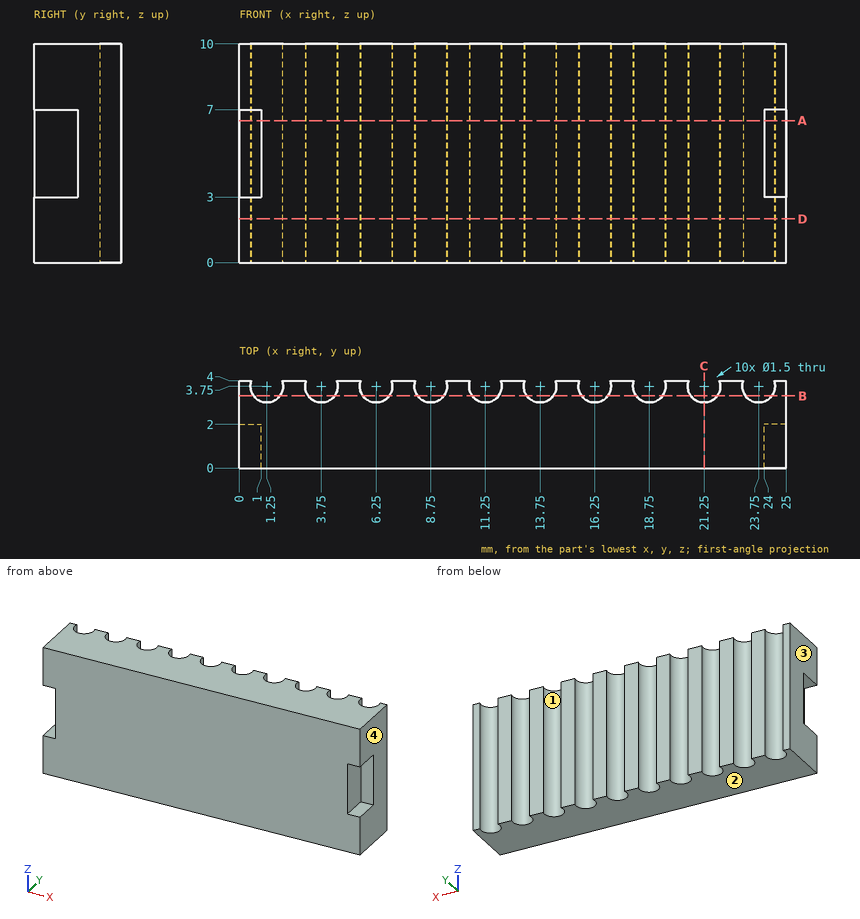
Can you work these out from the drawing? Everything is in mm from the part's minimum corner. Coordinates: 2 decimals unless noted, no trailing zeros. Write each loop counter-clockwise with the first axis right and the second up, starting at its lowest first coordinate (ties: lowest second). Pieces come first, ordered by that corner, then holes. Notation, with made-up numbers: (83.25, -18.5) -> (87.25, -18.5) arc R21 cw to (87.25, -0.5) -> close; hole circle Ø11 at (24.5, 20.25). An arc over 180 degrees is marked (long way). Write each question's results on one line, items separated by ' | '. Start each with the question number.
Q1. Imagine slicing it at A-A (z = 6.5). Write out the boundary of the cut face in (x, y), then the cut area to 3 significant figures.
Q2. Imagine slicing it at D-D (z = 2). Write out the boundary of the cut face in (x, y).
Q3. We'd pull the mould along X, two halves only. Please class the marked faces 1, 2, 3 and 4: +X half, -X half, draft (parallel to the pull), parting line (faces both ways), or undercut.
Q4. Imagine slicing it at B-B (y = 3.3). State how many separate pieces and enclosed holes the cut face has, then the cut area to 3 significant figures.
Q5. Imagine slicing it at C-C (x = 21.25). Write out the boundary of the cut face in (y, z).
Q6. If I drill on probe 1 along Y at (x, z) = (21.5, 1.5); probe 2 along Y at (x, z) = (11.75, 8.5), over which ranges is the centre line in solid material (lowest first)?
Taken from the geometry:
1) outline: (0, 2) -> (1, 2) -> (1, 0) -> (24, 0) -> (24, 2) -> (25, 2) -> (25, 4) -> (24.46, 4) arc R0.75 cw (long way) to (23.04, 4) -> (21.96, 4) arc R0.75 cw (long way) to (20.54, 4) -> (19.46, 4) arc R0.75 cw (long way) to (18.04, 4) -> (16.96, 4) arc R0.75 cw (long way) to (15.54, 4) -> (14.46, 4) arc R0.75 cw (long way) to (13.04, 4) -> (11.96, 4) arc R0.75 cw (long way) to (10.54, 4) -> (9.46, 4) arc R0.75 cw (long way) to (8.04, 4) -> (6.96, 4) arc R0.75 cw (long way) to (5.54, 4) -> (4.46, 4) arc R0.75 cw (long way) to (3.04, 4) -> (1.96, 4) arc R0.75 cw (long way) to (0.54, 4) -> (0, 4) -> close | area: 83.5 mm^2
2) outline: (0, 0) -> (25, 0) -> (25, 4) -> (24.46, 4) arc R0.75 cw (long way) to (23.04, 4) -> (21.96, 4) arc R0.75 cw (long way) to (20.54, 4) -> (19.46, 4) arc R0.75 cw (long way) to (18.04, 4) -> (16.96, 4) arc R0.75 cw (long way) to (15.54, 4) -> (14.46, 4) arc R0.75 cw (long way) to (13.04, 4) -> (11.96, 4) arc R0.75 cw (long way) to (10.54, 4) -> (9.46, 4) arc R0.75 cw (long way) to (8.04, 4) -> (6.96, 4) arc R0.75 cw (long way) to (5.54, 4) -> (4.46, 4) arc R0.75 cw (long way) to (3.04, 4) -> (1.96, 4) arc R0.75 cw (long way) to (0.54, 4) -> (0, 4) -> close
3) face 1: undercut | face 2: draft | face 3: -X half | face 4: +X half
4) separate pieces: 11 | enclosed holes: 0 | area: 130 mm^2
5) outline: (0, 0) -> (3, 0) -> (3, 10) -> (0, 10) -> close
6) probe 1: y = 0 to 3.04 | probe 2: y = 0 to 3.19
